Verification items for the finished model (mm, model axes). A direction names the side the tool comes from. Give positions to 0.01 mm unless a question says otherwise; leave off trailing zeros. Loops run counter-clockwise (first coordinate to the right, second up) from the corner with the lowest first, then second, coordinate; pieces in that order, holes last. Notation, with made-up numbers: (-6.75, -28) - (49.25, -28) arc R21 ccw to (49.25, -21) - close; hole circle Ø4 at (52, 81.25). An arc over 180 degrees is marked (long way). One line per item, written item: value. Start each with the question number.
1. Sectioned sample at D-D (z = 22.5). Record the cut outline in (x, y), plus the area to 3 significant figures.
2. Scan lines: L1, parallel to X at y = -2.5, z = 64; L2, parallel to X at y = -5.5, z = 11.5; L3, parallel to X at y = 3.8, z = -15.5. Record each from-to range of solid material in increasing order. Write a range as [from, to].
3. Mould release check, pull along X, two halves, no side actions. Record for faces 4 (the flat face through (-11, -21.056, 23)), 5 (the flat face through (-34, -14, 34)), 6 (the flat face through (-59, -14, 61)): pulls with the +X half, pulls with the -X half, needs draft (parallel to the pull), parting line crosses it, or undercut.
4. Sectioned sample at B-B (x = 0). Record the cut outline in (y, z), plus the area to 4 significant figures.
5. Gauge pin test, flat ends, axial feed: pin 1 (4.5 mm diameter, centred on x = 11, y = -25, fed in from -Z); pin 2 (3 mm diameter, centred on x = -12, y = -24, fed in from -Z); pin 3 (3 mm diameter, centred on y = -10, z = 15.5, fed in from -X). Record the tip position at first contact, or that the pin passes through.
6. Access from +Z, -Z, +X, -X, +Y, -Y to the whole of each face (thin tool, end or side, straight path). Record for faces 1 (the flat face through (-14.4, 0, -5)), 2 (the flat face through (-13.712, -22.548, 22.629)), 3 (the flat face through (32.17, -13.73, 44.31)).
7. Sectioned sample at C-C (z = 64.5). Record the cut outline in (x, y).
8. Sectioned sample at A-A (z = 0). Record the cut outline in (x, y), plus the area to 4 significant figures.
from build123d import *

# Parameters (mm, degrees)
SKETCH_6_W          = 42.3
SKETCH_6_H          = 42.3
SKETCH_6_R          = 1.6
SKETCH_6_R_2        = 15
EXTRUDE_1_DEPTH     = 5
SKETCH_7_R          = 4.1
EXTRUDE_5_DEPTH     = 38
EXTRUDE_START       = 38
SKETCH_7_7_R        = 4.1
EXTRUDE_7_DEPTH     = 38
SKETCH_7_8_R        = 4.1
EXTRUDE_8_DEPTH     = 38
SKETCH_12_W         = 2
SKETCH_12_H         = 44.3
EXTRUDE_11_DEPTH    = 38
SKETCH_14_W         = 44.3
SKETCH_14_H         = 2
EXTRUDE_12_DEPTH    = 38
SKETCH_15_W         = 2
SKETCH_15_H         = 42.3
EXTRUDE_13_DEPTH    = 38
SKETCH_17_W         = 122.95750499
SKETCH_17_H         = 7
CUT_EXTRUDE_1_DEPTH = 19
EXTRUDE_14_DEPTH    = 38
CUT_EXTRUDE_3_DEPTH = 3
SKETCH_22_R         = 1.5
CUT_EXTRUDE_4_DEPTH = 10


with BuildPart() as part:
    # 草图6 → 凸台-拉伸1 (new body)
    with BuildSketch(Plane(origin=(0, 0, 0), x_dir=(1, 0, 0), z_dir=(0, 1, 0))):
        Rectangle(SKETCH_6_W, SKETCH_6_H)
        with Locations(Location((15.5, 15.5, 0), (0, 0, 270))):
            Circle(SKETCH_6_R, mode=Mode.SUBTRACT)
        with Locations(Location((-15.5, 15.5, 0), (0, 0, 270))):
            Circle(SKETCH_6_R, mode=Mode.SUBTRACT)
        with Locations(Location((-15.5, -15.5, 0), (0, 0, 270))):
            Circle(SKETCH_6_R, mode=Mode.SUBTRACT)
        with Locations(Location((15.5, -15.5, 0), (0, 0, 270))):
            Circle(SKETCH_6_R, mode=Mode.SUBTRACT)
        with Locations(Location((0, 0, 0), (0, 0, 270))):
            Circle(SKETCH_6_R_2, mode=Mode.SUBTRACT)
    extrude(amount=EXTRUDE_1_DEPTH)

    # 草图7 → 凸台-拉伸5 (add)
    # profile 1 of 2: a face of its own
    with BuildSketch(Plane(origin=(0, 5, 0), x_dir=(1, 0, 0), z_dir=(0, 1, 0))):
        with BuildLine():
            Line((-41, -53.596295528), (-10.142654247, -21.15))
            Line((-10.142654247, -21.15), (-21.15, -21.15))
            Line((-21.15, -21.15), (-21.15, -10.142654247))
            Line((-21.15, -10.142654247), (-56.202269248, -43.478354795))
            ThreePointArc((-56.202269248, -43.478354795), (-58.271046585, -46.45179082), (-59, -50))
            Line((-59, -50), (-59, -73.238133914))
            Line((-59, -73.238133914), (-41, -73.238133914))
            Line((-41, -73.238133914), (-41, -53.596295528))
        make_face()
        with Locations(Location((-50, -64, 0), (0, 0, 270))):
            Circle(SKETCH_7_R, mode=Mode.SUBTRACT)
    # profile 2 of 2: a face of its own
    with BuildSketch(Plane(origin=(0, 5, 0), x_dir=(1, 0, 0), z_dir=(0, 1, 0))):
        with BuildLine():
            Line((21.15, -21.15), (10.142654247, -21.15))
            Line((10.142654247, -21.15), (41, -53.596295528))
            Line((41, -53.596295528), (41, -73.238133914))
            Line((41, -73.238133914), (59, -73.238133914))
            Line((59, -73.238133914), (59, -50))
            ThreePointArc((59, -50), (58.271046585, -46.45179082), (56.202269248, -43.478354795))
            Line((56.202269248, -43.478354795), (21.15, -10.142654247))
            Line((21.15, -10.142654247), (21.15, -21.15))
        make_face()
        with Locations(Location((50, -64, 0), (0, 0, 270))):
            Circle(SKETCH_7_R, mode=Mode.SUBTRACT)
    extrude(amount=-EXTRUDE_5_DEPTH)

    # 草图7<7> → 凸台-拉伸7 (add)
    with BuildSketch(Plane(origin=(0, 5, 0), x_dir=(1, 0, 0), z_dir=(0, 1, 0)).offset(EXTRUDE_START)):
        with Locations(Location((-50, -64, 0), (0, 0, 270))):
            Circle(SKETCH_7_7_R)
        with Locations(Location((50, -64, 0), (0, 0, 270))):
            Circle(SKETCH_7_7_R)
    extrude(amount=-EXTRUDE_7_DEPTH)


with BuildPart() as extrude_7_kept_piece:
    # of the separate pieces the step leaves, the one the design keeps (extrude_7_pieces_kept)
    add(part.part.solids().sort_by_distance((-10.142654247, 0, 21.15))[0])

    # 草图7<8> → 凸台-拉伸8 (add)
    with BuildSketch(Plane(origin=(0, 5, 0), x_dir=(1, 0, 0), z_dir=(0, 1, 0))):
        with Locations(Location((-50, -64, 0), (0, 0, 270))):
            Circle(SKETCH_7_8_R)
        with Locations(Location((50, -64, 0), (0, 0, 270))):
            Circle(SKETCH_7_8_R)
    extrude(amount=EXTRUDE_8_DEPTH)


with BuildPart() as extrude_8_kept_piece:
    # of the separate pieces the step leaves, the one the design keeps (extrude_8_pieces_kept)
    add(extrude_7_kept_piece.part.solids().sort_by_distance((-10.142654247, 0, 21.15))[0])

    # 草图12 → 凸台-拉伸11 (add)
    with BuildSketch(Plane(origin=(0, 5, 0), x_dir=(1, 0, 0), z_dir=(0, 1, 0))):
        with Locations((22.15, -1)):
            Rectangle(SKETCH_12_W, SKETCH_12_H)
    extrude(amount=-EXTRUDE_11_DEPTH)

    # 草图14 → 凸台-拉伸12 (add)
    with BuildSketch(Plane(origin=(0, 5, 0), x_dir=(1, 0, 0), z_dir=(0, 1, 0))):
        with Locations((-1, -22.15)):
            Rectangle(SKETCH_14_W, SKETCH_14_H)
    extrude(amount=-EXTRUDE_12_DEPTH)

    # 草图15 → 凸台-拉伸13 (add)
    with BuildSketch(Plane(origin=(0, 5, 0), x_dir=(1, 0, 0), z_dir=(0, 1, 0))):
        with Locations((-22.15, 0)):
            Rectangle(SKETCH_15_W, SKETCH_15_H)
    extrude(amount=-EXTRUDE_13_DEPTH)

    # 草图17 → 切除-拉伸1 (cut)
    with BuildSketch(Plane.XZ.offset(33)):
        with Locations((-0.358433095, 33.65)):
            Rectangle(SKETCH_17_W, SKETCH_17_H)
    extrude(amount=-CUT_EXTRUDE_1_DEPTH, mode=Mode.SUBTRACT)

    # 草图21 → 凸台-拉伸14 (add)
    with BuildSketch(Plane.XZ.offset(33)):
        Polygon((18.701909079, 30.15), (-18.701909079, 30.15), (-12.044710877, 23.15), (12.044710877, 23.15), align=None)
    extrude(amount=-EXTRUDE_14_DEPTH)

    # 草图20 → 切除-拉伸3 (cut)
    with BuildSketch(Plane(origin=(0, 0, 21.15), x_dir=(-1, 0, 0), z_dir=(0, 0, -1))):
        Polygon((-7.75, -24), (-9.45, -21.055513627), (-12.85, -21.055513627), (-14.55, -24), (-12.85, -26.944486373), (-9.45, -26.944486373), align=None)
        Polygon((14.55, -24), (12.85, -21.055513627), (9.45, -21.055513627), (7.75, -24), (9.45, -26.944486373), (12.85, -26.944486373), align=None)
    extrude(amount=-CUT_EXTRUDE_3_DEPTH, mode=Mode.SUBTRACT)

    # 草图22 → 切除-拉伸4 (cut)
    with BuildSketch(Plane(origin=(0, 0, 21.15), x_dir=(-1, 0, 0), z_dir=(0, 0, -1))):
        with Locations((11.15, -24)):
            Circle(SKETCH_22_R)
        with Locations((-11.15, -24)):
            Circle(SKETCH_22_R)
    extrude(amount=-CUT_EXTRUDE_4_DEPTH, mode=Mode.SUBTRACT)


solid = extrude_8_kept_piece.part
Results are:
1. outline: (-34.14, -33) - (34.14, -33) - (34.14, 5) - (-34.14, 5) - close; hole (-14.55, -24) - (-12.85, -26.94) - (-9.45, -26.94) - (-7.75, -24) - (-9.45, -21.06) - (-12.85, -21.06) - close; hole (7.75, -24) - (9.45, -26.94) - (12.85, -26.94) - (14.55, -24) - (12.85, -21.06) - (9.45, -21.06) - close
1. area: 2,530 mm^2
2. L1: x = [-59, -54.1], [-45.9, -41], [41, 45.9], [54.1, 59]
2. L2: x = [-23.15, -21.15], [21.15, 23.15]
2. L3: x = [-23.15, -17.1], [-13.9, 13.9], [17.1, 23.15]
3. face 4: undercut
3. face 5: needs draft
3. face 6: pulls with the -X half
4. outline: (-33, 21.15) - (0, 21.15) - (0, 15) - (5, 15) - (5, 30.15) - (-33, 30.15) - close; (0, -21.15) - (5, -21.15) - (5, -15) - (0, -15) - close
4. area: 403.5 mm^2
5. pin 1: stops at z = 21.15
5. pin 2: stops at z = 24.15
5. pin 3: stops at x = -28.36
6. face 1: -Z, -Y
6. face 2: -Z
6. face 3: +Z, +Y, -Y
7. outline: (-59, -33) - (-54.07, -33) - (-54.07, 5) - (-59, 5) - close; (-45.93, -33) - (-41, -33) - (-41, 5) - (-45.93, 5) - close; (41, -33) - (45.93, -33) - (45.93, 5) - (41, 5) - close; (54.07, -33) - (59, -33) - (59, 5) - (54.07, 5) - close
8. outline: (-23.15, -33) - (-21.15, -33) - (-21.15, 0) - (-15, 0) - (-15, 5) - (-23.15, 5) - close; (15, 0) - (21.15, 0) - (21.15, -33) - (23.15, -33) - (23.15, 5) - (15, 5) - close
8. area: 213.5 mm^2
